```python
from build123d import *

# Parameters (mm, degrees)
F0_W     = 8.636
F0_H     = 9.144
F0_R     = 4.191
F1_DEPTH = 3.048
F0_R_2   = 3.683
F2_DEPTH = 1.016
F3_DEPTH = 2.032


with BuildPart() as f1:
    # F0 (on Front) → F1 (new body)
    with BuildSketch(Plane.XZ):
        with Locations((0, -8.227191)):
            Rectangle(F0_W, F0_H)
        with Locations((0, -8.227191)):
            Circle(F0_R, mode=Mode.SUBTRACT)
    extrude(amount=F1_DEPTH)

    # F0 (on Front) → F2 (join)
    with BuildSketch(Plane.XZ):
        with Locations((0, -8.227191)):
            Rectangle(F0_W, F0_H)
        with Locations((0, -8.227191)):
            Circle(F0_R, mode=Mode.SUBTRACT)
        with Locations((0, -8.227191)):
            Circle(F0_R_2)
        with Locations((0, -8.227191)):
            Circle(F0_R)
        with Locations((0, -8.227191)):
            Circle(F0_R_2, mode=Mode.SUBTRACT)
    extrude(amount=-F2_DEPTH)

    # F0 (on Front) → F3 (join)
    with BuildSketch(Plane.XZ):
        with Locations((0, -8.227191)):
            Circle(F0_R_2)
    extrude(amount=-F3_DEPTH)


solid = f1.part
```
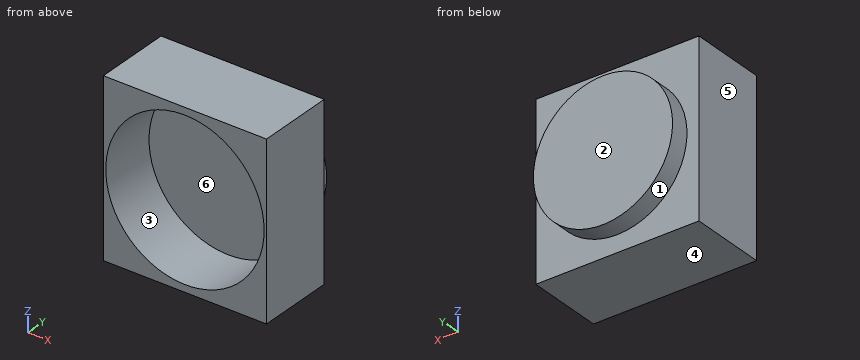
Design review of the part built by this model. Coordinates are the model's own, in mm. Face numbers are marked on the shaded views. A direction names the side the tool comes from. Give positions to 0.01 mm unless a question says otherwise; leave off trailing zeros. Order: outer loops, then holes, each group sorted by start corner. A loop starts at its lowest first (then second) coordinate and runs counter-clockwise, first axis right, second up. Notation, with made-up numbers: M -22,68.25 L -1,68.25 A19 ccw -1,72.25 Z; hole C -13.5,-33.5 d7. An arc over 180 degrees is marked long. One line per question, with ' | ' between items. Start each with the question number.
Q1. We need section A-A (x = 0). Write out the cut boundary in (y, z), plus the area to 3 significant figures.
Q2. The part is to be moulded in two halves that separate along Z. For the marked faces 4, 5 and 6, say which applies: +Z half, -Z half, draft (parallel to the pull), parting line (faces both ways), or undercut.
Q3. We need section B-B (y = -2.5). Write out the cut boundary in (x, z).
Q4. We need section C-C (z = -11). Write out the cut boundary in (x, y), plus the area to 3 significant figures.
Q5. For pin 1 Ø2 at (x, z) = (-1, -7.5) entering from -Y, flat-tipped, find the tip position at first contact; note if it passes through.
Q6. For L1, parallel to Z at x = 0, y = -1.15; L2, parallel to Y at x = 2, z = -8.25; L3, parallel to Y at x = -3.5, z = -11.5, list the stretches that pass through material, from the lowest coordinate up. Write a range as [from, to].
Q7. Machinability: for the marked faces 1, 2 and 3, which of the approach directions +Z, -Z, +X, -X, +Y, -Y give a long, thin tool a straight path to every point of the face, cutting with its end or side? Answer none if there is none.
Returned:
1) outline: M -3.05,-12.8 L 1.02,-12.8 L 1.02,-11.91 L 2.03,-11.91 L 2.03,-4.54 L 1.02,-4.54 L 1.02,-3.66 L -3.05,-3.66 L -3.05,-4.04 L 0,-4.04 L 0,-12.42 L -3.05,-12.42 Z | area: 19.1 mm2
2) face 4: -Z half | face 5: draft | face 6: undercut
3) outline: M -4.32,-12.8 L 4.32,-12.8 L 4.32,-3.66 L -4.32,-3.66 Z; hole C 0,-8.23 d8.38
4) outline: M -4.32,-3.05 L -3.14,-3.05 L -3.14,0 L 3.14,0 L 3.14,-3.05 L 4.32,-3.05 L 4.32,1.02 L 2.42,1.02 L 2.42,2.03 L -2.42,2.03 L -2.42,1.02 L -4.32,1.02 Z | area: 20.9 mm2
5) pin 1: y = 0
6) L1: [-12.8, -12.42], [-4.04, -3.66] | L2: [0, 2.03] | L3: [-3.05, 1.02]
7) face 1: +Y | face 2: +Z, -Z, +X, -X, +Y | face 3: -Y
